```python
from build123d import *

# Parameters (mm, degrees)
SKIZZE1_W                       = 498
SKIZZE1_H                       = 498
AUFSATZ_LINEAR_AUSTRAGEN1_DEPTH = 2
SCHNITT_LINEAR_AUSTRAGEN2_DEPTH = 2


with BuildPart() as part:
    # Skizze1 → Aufsatz-Linear austragen1 (new body)
    with BuildSketch(Plane(origin=(0, 0, 0), x_dir=(1, 0, 0), z_dir=(0, 1, 0))):
        Rectangle(SKIZZE1_W, SKIZZE1_H)
    extrude(amount=-AUFSATZ_LINEAR_AUSTRAGEN1_DEPTH)

    # Skizze3 → Schnitt-Linear austragen2 (cut)
    with BuildSketch(Plane.XZ.offset(2)):
        with BuildLine():
            ThreePointArc((-244, 244), (0, 3.66854455), (244, 244))
            ThreePointArc((244, 244), (101.068109219, -101.068109219), (-244, -244))
            Line((-244, -244), (-244, 244))
        make_face()
    extrude(amount=-SCHNITT_LINEAR_AUSTRAGEN2_DEPTH, mode=Mode.SUBTRACT)


solid = part.part
```
Design review of the part built by this model. Coordinates are the model's own, in mm. Round coordinates to 2 decimals unless told otherwise and drop trailing zeros. Write each loop counter-clockwise with the first axis right and the second up, starting at its lowest first coordinate (ties: lowest second). Pieces come first, ordered by that corner, then holes.
Item 1: We need section A-A on x = 0. Write out the cut boundary in (y, z).
Item 2: We need section C-C on z = -6. Write out the cut boundary in (x, y), and give its area (3 significant figures).
Item 3: For probe 1 along X at (y, z) = (-1.55, 208); probe 2 along X at (y, z) = (-0.3, 22); probe 3 along X at (y, z) = (-1.05, -1.5), list the stretches that pass through material, from the lowest coordinate up.
Item 4: Clearance check with a flat-ended pin moving along its axis: pin 1 Ø1.5 at (x, z) = (60, 139.5) entering from +Y. State where the tip first meets the part, or that it passes through.
Item 5: The part is to be moulded in two halves that separate along Z. For faces 1 (the cylindrical face through (104.841, -1.014, -97.253)), 2 (the flat face through (52, 0, 52)), say which applies: +Z half, -Z half, draft (parallel to the pull), parting line (faces both ways), or undercut.
Item 6: We need section D-D on z = 189. Write out the cut boundary in (x, y).
Item 7: We need section B-B on y = -0.75. Write out the cut boundary in (x, z), and give its area (3 significant figures).
Returned:
1. outline: (-2, -249) - (0, -249) - (0, -178.62) - (-2, -178.62) - close; (-2, 3.67) - (0, 3.67) - (0, 249) - (-2, 249) - close
2. outline: (-249, -2) - (-244, -2) - (-244, 0) - (-249, 0) - close; (175.1, -2) - (249, -2) - (249, 0) - (175.1, 0) - close
2. area: 158 mm2
3. probe 1: x = -249 to -244, -240.78 to 240.78, 242.67 to 249
3. probe 2: x = -249 to -244, -92.79 to 92.79, 190.58 to 249
3. probe 3: x = -249 to -244, 177.75 to 249
4. pin 1: stops at y = 0
5. face 1: undercut
5. face 2: draft
6. outline: (-249, -2) - (-244, -2) - (-244, 0) - (-249, 0) - close; (-236.86, -2) - (236.86, -2) - (236.86, 0) - (-236.86, 0) - close; (240.89, -2) - (249, -2) - (249, 0) - (240.89, 0) - close
7. outline: (-249, -249) - (249, -249) - (249, 249) - (-249, 249) - close; hole (-244, -244) arc R488 ccw to (244, 244) arc R244.03 cw to (-244, 244) - close
7. area: 153,000 mm2
